Work out the finished part from the listing and answer in its coordinate system (mm). A direction names the side the tool comes from. Round coordinates to 2 decimals unless told otherwise and drop trailing zeros. Loops run counter-clockwise (first coordinate to the right, second up) from the corner with the lowest first, then second, coordinate; pieces in that order, holes last.
```python
from build123d import *

# Parameters (mm, degrees)
SKETCH1_R           = 3.3
SKETCH1_R_2         = 0.889
BOSS_EXTRUDE1_DEPTH = 6.35
SKETCH3_W           = 6.5
SKETCH3_H           = 10.724019234
CUT_EXTRUDE2_DEPTH  = 2.85


with BuildPart() as part:
    # Sketch1 → Boss-Extrude1 (new body)
    with BuildSketch(Plane(origin=(0, 0, 0), x_dir=(1, 0, 0), z_dir=(0, 1, 0))):
        with BuildLine():
            Line((10, -7.2), (10, -75.857864376))
            Line((10, -75.857864376), (30, -100))
            Line((30, -100), (30, -180))
            ThreePointArc((30, -180), (0, -210), (-30, -180))
            Line((-30, -180), (-10, 0))
            ThreePointArc((-10, 0), (-2.709235972, 9.626008542), (8.532008089, 5.215825723))
            Line((8.532008089, 5.215825723), (75, 5.215825723))
            Line((75, 5.215825723), (150, 5.215825723))
            ThreePointArc((150, 5.215825723), (154.485699703, 3.357788069), (156.343737357, -1.127911635))
            Line((156.343737357, -1.127911635), (170, -87.2))
            Line((170, -87.2), (170, -127.2))
            ThreePointArc((170, -127.2), (150, -147.2), (130, -127.2))
            Line((130, -127.2), (130, -87.2))
            ThreePointArc((130, -87.2), (135.857864376, -73.057864376), (150, -67.2))
            Line((150, -67.2), (150, -7.2))
            Line((150, -7.2), (100, -7.2))
            Line((100, -7.2), (96, -3.2))
            Line((96, -3.2), (84, -3.2))
            Line((84, -3.2), (72, -3.2))
            Line((72, -3.2), (68, -7.2))
            Line((68, -7.2), (59, -7.2))
            Line((59, -7.2), (10, -7.2))
        make_face()
        with Locations(Location((0, 0, 0), (0, 0, 270))):
            Circle(SKETCH1_R, mode=Mode.SUBTRACT)
        with Locations(Location((0, -180, 0), (0, 0, 270))):
            Circle(SKETCH1_R, mode=Mode.SUBTRACT)
        with Locations(Location((150, -87.2, 0), (0, 0, 270))):
            Circle(SKETCH1_R, mode=Mode.SUBTRACT)
        with Locations(Location((84, -1.5, 0), (0, 0, 270))):
            Circle(SKETCH1_R_2, mode=Mode.SUBTRACT)
        with Locations(Location((84, 3.216, 0), (0, 0, 270))):
            Circle(SKETCH1_R_2, mode=Mode.SUBTRACT)
        with Locations(Location((150, -127.2, 0), (0, 0, 270))):
            Circle(SKETCH1_R, mode=Mode.SUBTRACT)
        with Locations(Location((0, -160, 0), (0, 0, 270))):
            Circle(SKETCH1_R, mode=Mode.SUBTRACT)
        with Locations(Location((0, -140, 0), (0, 0, 270))):
            Circle(SKETCH1_R, mode=Mode.SUBTRACT)
    extrude(amount=BOSS_EXTRUDE1_DEPTH)

    # Sketch3 → Cut-Extrude2 (cut)
    with BuildSketch(Plane(origin=(0, 6.35, 0), x_dir=(1, 0, 0), z_dir=(0, 1, 0))):
        with Locations((84, 0.476239432)):
            Rectangle(SKETCH3_W, SKETCH3_H)
    extrude(amount=-CUT_EXTRUDE2_DEPTH, mode=Mode.SUBTRACT)


solid = part.part
```
1. Which of the six approach directions +Z, -Z, +X, -X, +Y, -Y give full straight-line access (tool end or side, diameter ignored) to faces 1 (the face through (154.436, 3.131, -3.407)), 2 (the face through (19.86, 3.13, 87.76)), 3 (the face through (84, 3, 3.2))?
Answer key:
face 1: -Z, +X, +Y, -Y
face 2: +Y, -Y
face 3: +Z, +Y, -Y
2. Find section A-A (x = 0). Write down the section's boundary in (y, z), then the cut area to 3 significant figures.
Answer key:
outline: (0, -10) - (6.35, -10) - (6.35, -3.3) - (0, -3.3) - close; (0, 3.3) - (6.35, 3.3) - (6.35, 136.7) - (0, 136.7) - close; (0, 143.3) - (6.35, 143.3) - (6.35, 156.7) - (0, 156.7) - close; (0, 163.3) - (6.35, 163.3) - (6.35, 176.7) - (0, 176.7) - close; (0, 183.3) - (6.35, 183.3) - (6.35, 210) - (0, 210) - close
area: 1,230 mm2
3. Find section B-B (y = 1). Give the number of separate pieces and of enclosed holes in the cut face, then the cut area to 3 significant figures.
Answer key:
separate pieces: 1
enclosed holes: 8
area: 13,900 mm2
4. Find section D-D (x = 60). Write down the section's boundary in (y, z), then the cut area to 3 significant figures.
Answer key:
outline: (0, -5.22) - (6.35, -5.22) - (6.35, 7.2) - (0, 7.2) - close
area: 78.8 mm2
5. Determine the mould class of faces 4 (the face through (-2.883, 3.131, -9.575)), 5 (the face through (153.27, 3.13, 126.77)), 6 (the face through (2.23, 3.13, 137.57)), 7 (the face through (144, 6.35, 71)) for opening direction Z: +Z half, -Z half, draft (parallel to the pull), parting line (faces both ways), or undercut.
Answer key:
face 4: -Z half
face 5: undercut
face 6: undercut
face 7: draft
6. Find section C-C (z = 160). Write down the section's boundary in (x, y), then the cut area to 3 significant figures.
Answer key:
outline: (-27.78, 0) - (-3.3, 0) - (-3.3, 6.35) - (-27.78, 6.35) - close; (3.3, 0) - (30, 0) - (30, 6.35) - (3.3, 6.35) - close
area: 325 mm2
7. Consider probe 1 along X at (y, z) = (5, 127.2); probe 2 along Z at (x, y) = (84, 1.75) (3 decimals); probe 3 along X at (y, z) = (3.25, 124.5). Determine where each line is inside the solid, lowest interval first.
Answer key:
probe 1: x = -24.13 to 30, 130 to 146.7, 153.3 to 170
probe 2: z = -5.216 to -4.105, -2.327 to 0.611, 2.389 to 3.2
probe 3: x = -23.83 to 30, 130 to 148.1, 151.9 to 170
8. Given pin 1 (1.5 mm diameter, centred on y = 5, z = 159.5, fed in from -X); pin 2 (1.5 mm diameter, centred on x = -8.5, y = 3.5, fed in from +Z); pin 3 (3 mm diameter, centred on x = 44.5, y = 2.5, fed in from +Z); pin 4 (5.5 mm diameter, centred on x = 150, z = 87.2, fed in from +Y), each flat-ended and moving along its own axis, determine where each tip first touches the part or whether it passes through.
Answer key:
pin 1: stops at x = -27.81
pin 2: stops at z = 208.98
pin 3: stops at z = 7.2
pin 4: passes through
